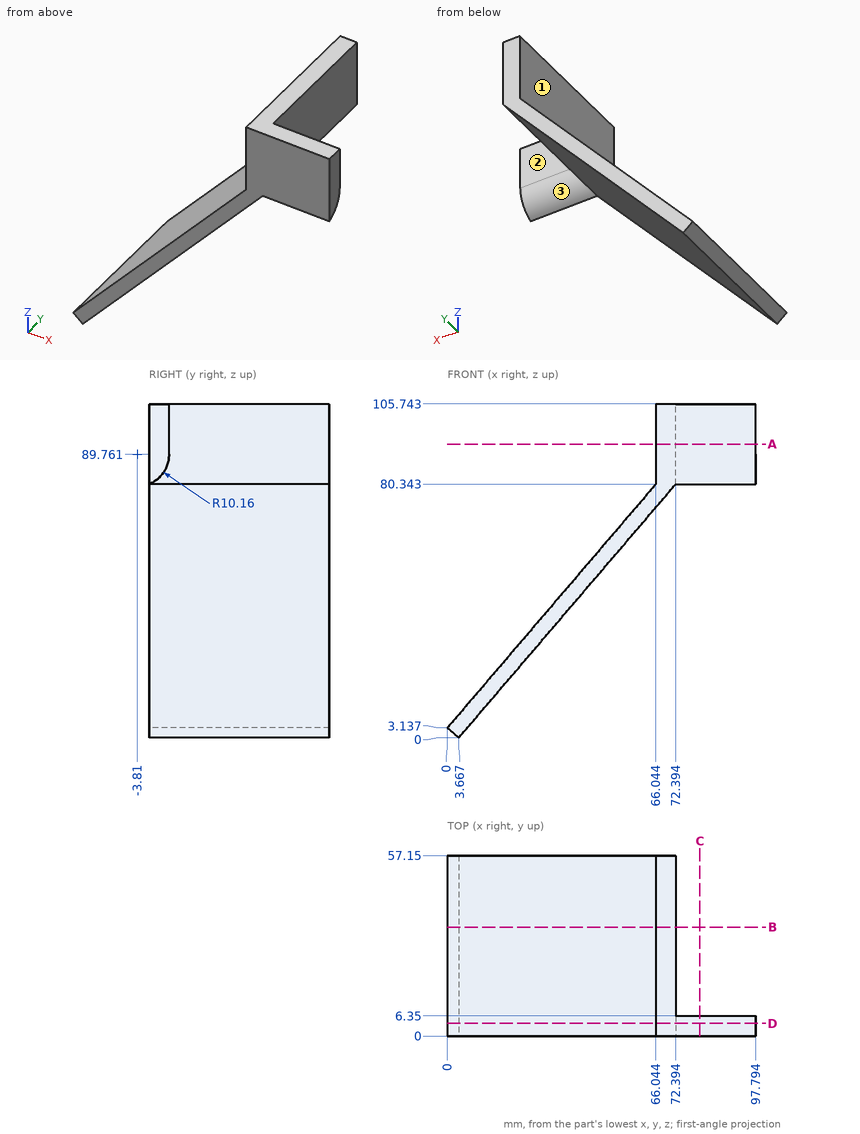
Geometry check sheet. Reference: drawing and pictorial views, mm from the part's lowest x, y, z. A direction names the side the tool comes from. Give positions to 0.01 mm unless a question says otherwise; leave off trailing zeros. Order: outer loops, then holes, each group sorted by start corner. A loop starts at its lowest first (then second) coordinate and runs counter-clockwise, first axis right, second up. Notation, with made-up numbers: (-39.5, 11.25) -> (5.5, 11.25) arc R22 cw to (5.5, 31.25) -> close; hole circle Ø2 at (-26.5, 33). An arc over 180 degrees is marked (long way). Use CSV: the item, a comma, the result in double quotes. Start each with the question number.
1) Sectioned sample at D-D, the plane y = 4. Record the boundary of the cut face in (x, z).
2) Set-up check for the marked faces 1, 2 and 3: record each of +Z, -Z, +X, -X, +Y, -Y from which the full face is reachable in a straight line by a thin tool's end or side.
3) Sectioned sample at C-C, the plane x = 80. Record the boundary of the cut face in (y, z), plus the area to 3 significant figures.
4) Sectioned sample at B-B, the plane y = 34.5. Record the boundary of the cut face in (x, z).
5) Material ranges on line 1 (X direction, y = 21.5, z = 83.5); line 2 (X direction, y = 24, z = 76); line 3 (Z direction, x = 41, y = 23) (1 decimal), recorded low to high. Write a range as from..to.
6) Sectioned sample at A-A, the plane z = 93. Record the boundary of the cut face in (x, y).
7) Go/stop test with flat-tipped pins: P1, Ø6, axis at y = 24, z = 93, coming from the +X side; P2, Ø7.5, axis at y = 28, z = 93.5, coming from the -X side; P3, Ø10, axis at y = 45.5, z = 63, coming from the +X side (1 decimal). Record where each tip stops, or that it passes through.
Recorded:
1,outline,"(0, 3.14) -> (3.67, 0) -> (72.39, 80.34) -> (72.39, 83.26) -> (97.79, 83.26) -> (97.79, 105.74) -> (66.04, 105.74) -> (66.04, 80.34) -> close"
2,face 1,"+Z, -X, +Y, -Y"
2,face 2,"+Z, -Z, +X, +Y"
2,face 3,"-Z, +X, +Y"
3,outline,"(0, 80.34) arc R10.16 ccw to (6.35, 89.76) -> (6.35, 105.74) -> (0, 105.74) -> close"
3,area,"145 mm2"
4,outline,"(0, 3.14) -> (3.67, 0) -> (72.39, 80.34) -> (72.39, 105.74) -> (66.04, 105.74) -> (66.04, 80.34) -> close"
5,line 1,"66.04..72.39"
5,line 2,"62.33..68.68"
5,line 3,"43.6..51.1"
6,outline,"(66.04, 0) -> (97.79, 0) -> (97.79, 6.35) -> (72.39, 6.35) -> (72.39, 57.15) -> (66.04, 57.15) -> close"
7,P1,"x = 72.39"
7,P2,"x = 66.04"
7,P3,"x = 61.8"
